Answer from the drawing. Dimensions are ordinates in mm from the lowest x, y and z of the part. A direction names the side the tool comes from. Coordinates: 2 decimals unless noted, no trailing zeros. Write each loop counter-clockwise with the first axis right and the second up, starting at its lowest first coordinate (ties: lowest second). Pieces come first, ordered by that corner, then holes. Notation, with made-up numbers: (-36, -30) -> (-13, -30) arc R22 cw to (-13, -2) -> close; hole circle Ø9 at (39, 33.25). An arc over 180 degrees is marked (long way). One line per item, written item: value. Start each with the question number.
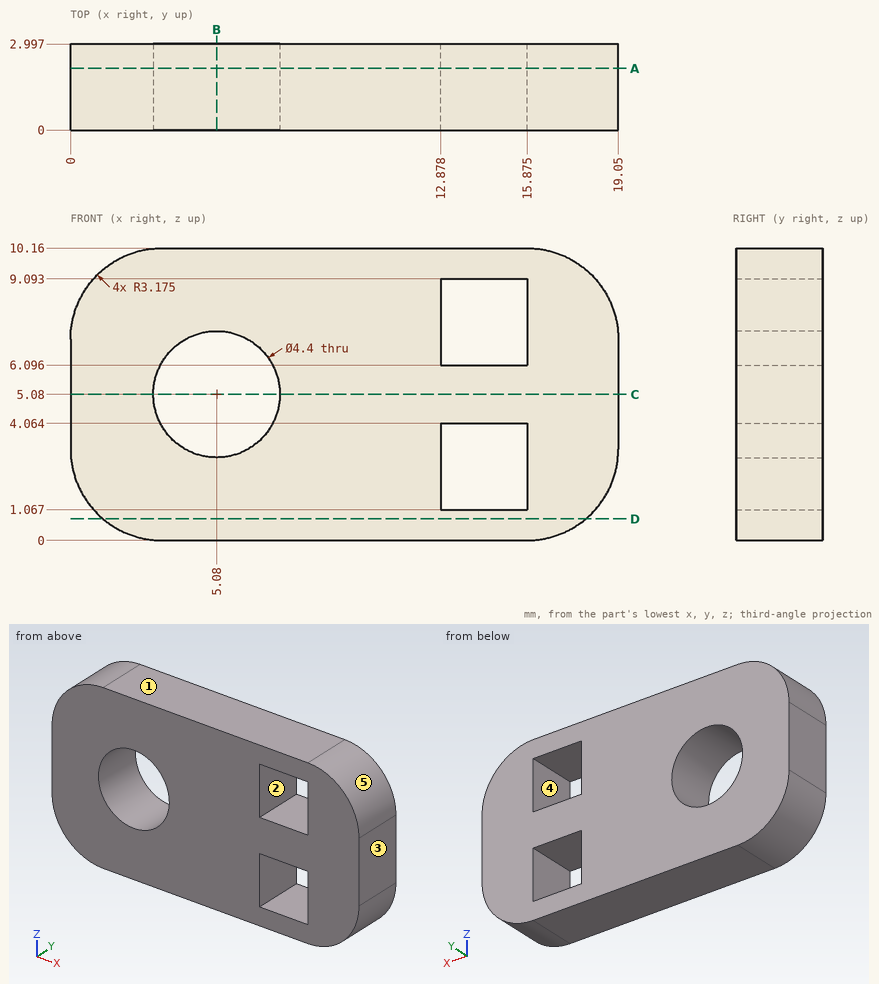
1. For a pull along X with two mould halves and no side action, classify the marked faces 1, 2 and 3 as +X half, -X half, draft (parallel to the pull), parting line (faces both ways), or undercut.
2. A cutting plane is placed at C-C on z = 5.08. Give the vertices of the cut face in (x, y), then the cut area to 3 significant figures.
3. A cutting plane is placed at D-D on z = 0.75. Give the vertices of the cut face in (x, y).
4. Find the intervals of material crossed by probe 1 along Z at (x, y) = (15, 1.35); probe 2 along X at (y, z) = (1.65, 5.08); probe 3 along X at (y, z) = (2.15, 1.5) (1 decimal), in increasing order. Write a range as from..to.
5. A tool of negligible diameter and unlimited length cuts with its end or side. For the marked faces 4 and 5, from which of +Z, -Z, +X, -X, +Y, -Y can it reach the whole face along a straight path? Write none if from no direction.
6. A cutting plane is placed at B-B on x = 5.08. Give the vertices of the cut face in (y, z).
7. A cutting plane is placed at A-A on y = 2.15. Count the separate pieces of the cut face and the enclosed holes in it, then the cut area to 3 significant figures.
Derived:
1. face 1: draft
1. face 2: undercut
1. face 3: +X half
2. outline: (0, 0) -> (2.88, 0) -> (2.88, 3) -> (0, 3) -> close; (7.28, 0) -> (19.05, 0) -> (19.05, 3) -> (7.28, 3) -> close
2. area: 43.9 mm2
3. outline: (1.13, 0) -> (17.92, 0) -> (17.92, 3) -> (1.13, 3) -> close
4. probe 1: z = 0..1.07, 4.06..6.1, 9.09..10.16
4. probe 2: x = 0..2.88, 7.28..19.05
4. probe 3: x = 0.5..12.9, 15.9..18.6
5. face 4: +Y, -Y
5. face 5: +Z, +X, +Y, -Y
6. outline: (0, 0) -> (3, 0) -> (3, 2.88) -> (0, 2.88) -> close; (0, 7.28) -> (3, 7.28) -> (3, 10.16) -> (0, 10.16) -> close
7. separate pieces: 1
7. enclosed holes: 3
7. area: 152 mm2
